Autodesk Inventor part; units mm, degrees
ref_plane "YZ Plane" through (0, 0, 0) normal (1, 0, 0) x (0, 1, 0)
ref_plane "XZ Plane" through (0, 0, 0) normal (0, 1, 0) x (-1, 0, 0)
ref_plane "XY Plane" through (0, 0, 0) normal (0, 0, 1) x (1, 0, 0)
sketch "Эскиз1" plane through (0, 0, 0) normal (0, 1, 0) x (-1, 0, 0)
  line L0 (50, -40) -> (-50, -40)
  line L1 (-50, -40) -> (-50, 40)
  line L2 (-50, 40) -> (50, 40)
  line L3 (50, 40) -> (50, -40)
  line L4 (50, -40) -> (-50, 40) construction
  line L5 (-50, -40) -> (50, 40) construction
  line L6 (21.6, -30) -> (-21.6, -30)
  line L7 (-21.6, -30) -> (-21.6, -6.9)
  line L8 (-21.6, -6.9) -> (21.6, -6.9)
  line L9 (21.6, -6.9) -> (21.6, -30)
  line L10 (-53, -43) -> (53, -43)
  line L11 (53, -43) -> (53, 43)
  line L12 (53, 43) -> (-53, 43)
  line L13 (-53, 43) -> (-53, -43)
  line L14 (53, 43) -> (68, 43)
  line L15 (68, 43) -> (68, -43)
  line L16 (68, -43) -> (53, -43)
  line L17 (53, -43) -> (53, 43)
  line L18 (-53, -43) -> (68, -43)
  line L19 (68, -43) -> (68, 43)
  line L20 (68, 43) -> (-53, 43)
  line L21 (-53, 43) -> (-53, -43)
  line L22 (0, -40) -> (0, 40)
  circle A0 centre (-30, 20) radius 5
  circle A1 centre (-30, 20) radius 7
  line L23 (-30, 20) -> (-30, 40)
  line L24 (-28, 30.5826) -> (-32, 30.5826)
  line L25 (-32, 30.5826) -> (-32, 24.5826)
  line L26 (-32, 24.5826) -> (-28, 24.5826)
  line L27 (-28, 24.5826) -> (-28, 30.5826)
  line L28 (-28, 30.5826) -> (-32, 24.5826) construction
  line L29 (-32, 30.5826) -> (-28, 24.5826) construction
  line L30 (-34, 22.5826) -> (-34, 32.5826)
  line L31 (-34, 32.5826) -> (-26, 32.5826)
  line L32 (-26, 32.5826) -> (-26, 22.5826)
  line L33 (-26, 22.5826) -> (-34, 22.5826)
  line L34 (-28, 30.5826) -> (-32, 30.5826)
  line L35 (-32, 30.5826) -> (-32, 32.5826)
  line L36 (-32, 32.5826) -> (-28, 32.5826)
  line L37 (-28, 32.5826) -> (-28, 30.5826)
  line L38 (-55.5, -45.5) -> (70.5, -45.5)
  line L39 (70.5, -45.5) -> (70.5, 45.5)
  line L40 (-55.5, -45.5) -> (-55.5, 45.5)
  line L41 (-55.5, 45.5) -> (70.5, 45.5)
  point P0 (0, 0)
  point P1 (0, -30)
  point P2 (-30, 27.5826)
  point P3 (53, -43)
  point P4 (-26, 25.7446)
  point P5 (-34, 25.7446)
  point P6 (53, -43)
  dimension "d7" = 10
  dimension "d0" = 100
  dimension "d1" = 80
  dimension "d2" = 43.2
  dimension "d3" = 23.1
  dimension "d4" = 3
  dimension "d5" = 15
  dimension "d6" = 10
  dimension "d8" = 2
  dimension "d9" = 20
  dimension "d10" = 20
  dimension "d11" = 4
  dimension "d12" = 6
  dimension "d13" = 2
  dimension "d22" = 2.5
  dimension "d23" = 2.5
extrude "Выдавливание1" add sketch "Эскиз1" along normal blind 2.5 contours L0 L22 L6 L9 L8 L2 L3 | L0 L1 L2 L22 L8 L7 L6 | L13 L12 L11 L10 | L11 L14 L15 L16 | A0 L30 L33 L32 | L32 L33 L23 L26 A0 | A0 L26 L23 L33 L30 | L26 L23 A0 | A0 L23 A1 L27 | L25 A1 L23 A0 | A0 L23 L26 | A1 L23 L24 L27 | L25 L24 L23 A1 | L24 L23 L31 L37 | L35 L31 L23 L24 | L40 L41 L39 L38
fillet "Сопряжение1" radius 5 4 edges at (26, 1.25, 25.7446) (28, 1.25, 24.5826) (32, 1.25, 24.5826) (34, 1.25, 25.7446)
fillet "Сопряжение2" radius 1 4 edges at (26, 1.25, 32.5826) (28, 1.25, 32.5826) (32, 1.25, 32.5826) (34, 1.25, 32.5826)
sketch "Эскиз2" plane through (0, 0, 0) normal (0, -1, 0) x (1, 0, 0)
  line L0 (-21.6, -30) -> (21.6, -30)
  line L1 (-21.6, -6.9) -> (-21.6, -30)
  line L2 (21.6, -6.9) -> (-21.6, -6.9)
  line L3 (21.6, -30) -> (21.6, -6.9)
  arc A0 (34, 27.9373) -> (35.25, 24.6301) centre (39, 27.9373) ccw
  arc A1 (24.75, 24.6301) -> (35.25, 24.6301) centre (30, 20) ccw
  arc A2 (24.75, 24.6301) -> (26, 27.9373) centre (21, 27.9373) ccw
  line L4 (26, 31.5826) -> (26, 27.9373)
  arc A3 (28, 31.5826) -> (26, 31.5826) centre (27, 31.5826) ccw
  line L5 (28, 27.1414) -> (28, 31.5826)
  arc A4 (26.5, 23.5707) -> (28, 27.1414) centre (23, 27.1414) ccw
  arc A5 (26.5, 23.5707) -> (33.5, 23.5707) centre (30, 20) ccw
  arc A6 (32, 27.1414) -> (33.5, 23.5707) centre (37, 27.1414) ccw
  line L6 (32, 31.5826) -> (32, 27.1414)
  arc A7 (34, 31.5826) -> (32, 31.5826) centre (33, 31.5826) ccw
  line L7 (34, 27.9373) -> (34, 31.5826)
  circle A8 centre (30, 20) radius 2.5
  point P0 (0, 0)
  dimension "d18" = 5
extrude "Выдавливание2" add sketch "Эскиз2" along normal blind 2.5 contours A8
fillet "Сопряжение3" radius 2 1 edges at (27.5, 0, 20)
sketch "Эскиз3" plane through (0, 0, 0) normal (0, -1, 0) x (1, 0, 0)
  arc A0 (34, 27.9373) -> (35.25, 24.6301) centre (39, 27.9373) ccw
  arc A1 (24.75, 24.6301) -> (35.25, 24.6301) centre (30, 20) ccw
  arc A2 (24.75, 24.6301) -> (26, 27.9373) centre (21, 27.9373) ccw
  line L0 (26, 31.5826) -> (26, 27.9373)
  arc A3 (28, 31.5826) -> (26, 31.5826) centre (27, 31.5826) ccw
  line L1 (28, 27.1414) -> (28, 31.5826)
  arc A4 (26.5, 23.5707) -> (28, 27.1414) centre (23, 27.1414) ccw
  arc A5 (26.5, 23.5707) -> (33.5, 23.5707) centre (30, 20) ccw
  arc A6 (32, 27.1414) -> (33.5, 23.5707) centre (37, 27.1414) ccw
  line L2 (32, 31.5826) -> (32, 27.1414)
  arc A7 (34, 31.5826) -> (32, 31.5826) centre (33, 31.5826) ccw
  line L3 (34, 27.9373) -> (34, 31.5826)
  line L4 (-21.6, -30) -> (21.6, -30)
  line L5 (-21.6, -6.9) -> (-21.6, -30)
  line L6 (21.6, -6.9) -> (-21.6, -6.9)
  line L7 (21.6, -30) -> (21.6, -6.9)
  circle A8 centre (30, 20) radius 4.5
  line L8 (55.5, -45.5) -> (-70.5, -45.5)
  line L9 (55.5, 45.5) -> (55.5, -45.5)
  line L10 (-70.5, 45.5) -> (55.5, 45.5)
  line L11 (-70.5, -45.5) -> (-70.5, 45.5)
  arc A9 (34, 27.9373) -> (35.25, 24.6301) centre (39, 27.9373) ccw
  arc A10 (24.75, 24.6301) -> (35.25, 24.6301) centre (30, 20) ccw
  arc A11 (24.75, 24.6301) -> (26, 27.9373) centre (21, 27.9373) ccw
  line L12 (26, 31.5826) -> (26, 27.9373)
  arc A12 (28, 31.5826) -> (26, 31.5826) centre (27, 31.5826) ccw
  line L13 (28, 27.1414) -> (28, 31.5826)
  arc A13 (26.5, 23.5707) -> (28, 27.1414) centre (23, 27.1414) ccw
  arc A14 (26.5, 23.5707) -> (33.5, 23.5707) centre (30, 20) ccw
  arc A15 (32, 27.1414) -> (33.5, 23.5707) centre (37, 27.1414) ccw
  line L14 (32, 31.5826) -> (32, 27.1414)
  arc A16 (34, 31.5826) -> (32, 31.5826) centre (33, 31.5826) ccw
  line L15 (34, 27.9373) -> (34, 31.5826)
  line L16 (-21.6, -30) -> (21.6, -30)
  line L17 (-21.6, -6.9) -> (-21.6, -30)
  line L18 (21.6, -6.9) -> (-21.6, -6.9)
  line L19 (21.6, -30) -> (21.6, -6.9)
  circle A17 centre (30, 20) radius 4.5
  line L20 (53, 43) -> (53, -43)
  line L21 (53, -43) -> (-68, -43)
  line L22 (-68, -43) -> (-68, 43)
  line L23 (-68, 43) -> (53, 43)
  dimension "d28" = 2.5
extrude "Выдавливание3" add sketch "Эскиз3" along normal blind 24.04 contours L8 L11 L10 L9
sketch "Эскиз4" plane through (-70.5, 2.5, -45.5) normal (-1, 0, 0) x (0, 0, 1)
  line L0 (91, -26.54) -> (91, 0)
  line L1 (0, 0) -> (91, 0)
  line L2 (0, -26.54) -> (0, 0)
  line L3 (91, -26.54) -> (0, -26.54)
  line L4 (0, 0) -> (0, -26.54)
  line L5 (0, -13.27) -> (-40, -13.27)
  circle A0 centre (-40, -13.27) radius 40
  line L6 (0, -26.54) -> (0, 0)
  line L7 (0, -26.54) -> (-2.2653, -26.54)
  line L8 (-2.2653, -26.54) -> (-2.2653, 0)
  line L9 (-2.2653, 0) -> (0, 0)
  line L10 (0, 0) -> (0, -26.54)
  line L11 (0, 0) -> (91, 0)
  point P0 (45.5, -2.5)
  point P1 (-2.2653, -26.54)
  dimension "d29" = 80
extrude "Выдавливание4" add sketch "Эскиз4" against normal up to surface (126 mm away) contours L7 A0 L2 | L2 A0 L9
sketch "Эскиз5" plane through (-70.5, -24.04, 45.5) normal (-1, 0, 0) x (0, 0, 1)
  line L0 (0, 0) -> (0, 26.54)
  line L1 (0, 26.54) -> (-93.2653, 26.54)
  arc A0 (-93.2653, 0) -> (-93.2653, 26.54) centre (-131, 13.27) ccw
  line L2 (0, 0) -> (-93.2653, 0)
  circle A1 centre (-131, 13.27) radius 40
  circle A2 centre (-131, 13.27) radius 36
  line L3 (-93.2653, 0) -> (-97.535, 0)
  arc A3 (-93.2653, 0) -> (-93.2653, 26.54) centre (-131, 13.27) ccw
  line L4 (-93.2653, 26.54) -> (-97.535, 26.54)
  point P0 (-45.5, 24.04)
  dimension "d32" = 4
extrude "Выдавливание5" add sketch "Эскиз5" against normal blind 4 contours L3 A2 L4 A0
sketch "Эскиз6" plane through (-70.5, -24.04, 45.5) normal (-1, 0, 0) x (0, 0, 1)
  line L0 (-2.5, 24.04) -> (-88.5, 24.04)
  line L1 (-2.5, 24.04) -> (-2.5, 0)
  line L2 (-88.5, 0) -> (-2.5, 0)
  line L3 (-88.5, 24.04) -> (-88.5, 0)
  line L4 (-88.5, 24.04) -> (-88.5, 0)
  line L5 (-88.5, 12.02) -> (-2.5, 12.02)
  line L6 (-2.5, 24.04) -> (-2.5, 0)
  line L7 (-10.5, 9.27) -> (-80.5, 9.27)
  line L8 (-80.5, 9.27) -> (-80.5, 14.77)
  line L9 (-80.5, 14.77) -> (-10.5, 14.77)
  line L10 (-10.5, 14.77) -> (-10.5, 9.27)
  line L11 (-10.5, 9.27) -> (-80.5, 14.77) construction
  line L12 (-80.5, 9.27) -> (-10.5, 14.77) construction
  point P0 (-45.5, 24.04)
  point P1 (-45.5, 12.02)
  dimension "d35" = 70
  dimension "d36" = 5.5
extrude "Выдавливание6" cut sketch "Эскиз6" against normal blind 4 contours L10 L7 L8 L5 | L5 L8 L9 L10
properties part number "tacho_base"
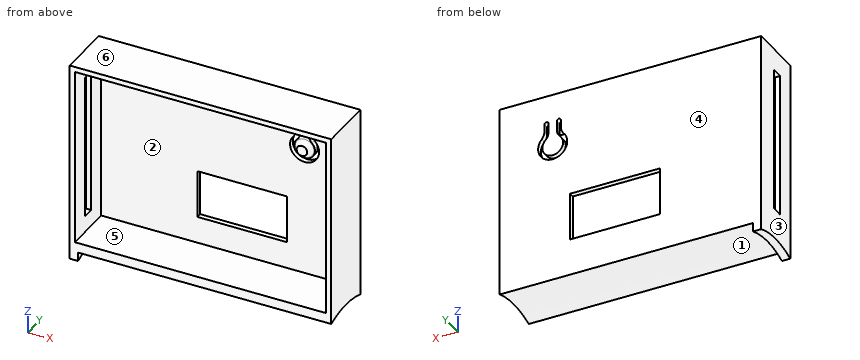
Geometry: final body of the model. Coordinates: model frame, mm. Face numbers are marked on the shaded views. A direction names the side the tool comes from. Round coordinates to 2 decimals unless told otherwise and drop trailing zeros. Order: outer loops, then holes, each group sorted by start corner. A loop starts at its lowest first (then second) coordinate and runs counter-clockwise, first axis right, second up. Notation, with made-up numbers: (83.25, -29) - (119.25, -29) arc R5 ccw to (119.25, -23) - close; hole circle Ø2 at (0, 84). An arc over 180 degrees is marked (long way). Use CSV: the item, a comma, the result in double quotes. Start each with the question number.
Q1. Section query A-A (z = 20). Return loops of the section in (x, y), and give its area (3 significant figures).
Q2. Section query D-D (y = -5.5). Return loops of the section in (x, z).
Q3. Material intervals for line 1 along X through (y, z) = (1.65, 20); line 2 along X through (y, z) = (-20.25, -11); line 3 along Z through (x, y) = (38.5, -11.25), sorted ascending. Write a range as from..to.
Q4. Access query for the marked faces 1, 2 and 3. Directions: +Z, -Z, +X, -X, +Y, -Y. A direction counts if a zero-diameter tool reaches every point of the face in a straight line with its end or side. Return the directions, or none.
Q5. Section query B-B (z = -22.5). Return loops of the section in (x, y).
Q6. First-contact query: pin 1 (3.5 mm diameter, centred on y = -6, z = -50, fed in from +X); pin 2 (10 mm diameter, centred on x = 39.5, z = -14.5, fed in from -Y); pin 3 (18 mm diameter, centred on x = 30, z = 20, fed in from -Y). Flat tips, straight axial feed; report the tip coordinate or a pass-through.
Q7. Mould query, pull axis Z, two halves, no side actions, for the marked faces 4, 5 and 6. Classes: +Z half, -Z half, draft (parallel to the pull), parting line (faces both ways), or undercut.
Q8. Section query C-C (x = 30). Return loops of the section in (y, z), and give its area (3 significant figures).
Result set:
1,outline,"(-70.5, -24.04) - (-68, -24.04) - (-68, -14.77) - (-70.5, -14.77) - close; (-70.5, -9.27) - (-68, -9.27) - (-68, 0) - (23, 0) - (23, 2.5) - (-70.5, 2.5) - close; (25, 0) - (25.5, 0) arc R2 cw to (27.5, -2) - (27.5, -2.5) - (32.5, -2.5) - (32.5, -2) arc R2 cw to (34.5, 0) - (35, 0) - (35, 2.5) - (25, 2.5) - close; (37, 0) - (53, 0) - (53, -24.04) - (55.5, -24.04) - (55.5, 2.5) - (37, 2.5) - close"
1,area,"426 mm2"
2,outline,"(-70.5, -49.89) - (-66.5, -49.89) - (-66.5, -45.85) - (55.5, -45.85) - (55.5, 45.5) - (-70.5, 45.5) - close; hole (-68, -43) - (53, -43) - (53, 43) - (-68, 43) - close"
3,line 1,"x = -70.5..23, 25..35, 37..55.5"
3,line 2,"x = -70.5..-68, 53..55.5"
3,line 3,"z = -45.5..-43, 43..45.5"
4,face 1,"-Z, +X"
4,face 2,"-Y"
4,face 3,"+Z, -Z, -X, +Y, -Y"
5,outline,"(-70.5, -24.04) - (-68, -24.04) - (-68, -14.77) - (-70.5, -14.77) - close; (-70.5, -9.27) - (-68, -9.27) - (-68, 0) - (-21.6, 0) - (-21.6, 2.5) - (-70.5, 2.5) - close; (21.6, 0) - (53, 0) - (53, -24.04) - (55.5, -24.04) - (55.5, 2.5) - (21.6, 2.5) - close"
6,pin 1,"stops at x = -66.5"
6,pin 2,"stops at y = 0"
6,pin 3,"stops at y = -2.5"
7,face 4,"draft"
7,face 5,"undercut"
7,face 6,"+Z half"
8,outline,"(-24.04, -47.77) arc R40 cw to (2.5, -47.77) - (2.5, 13) - (0, 13) - (0, -43) - (-24.04, -43) - close; (-24.04, 43) - (0, 43) - (0, 24.5) arc R2 cw to (-2, 22.5) - (-2.5, 22.5) - (-2.5, 17.5) - (-2, 17.5) arc R2 cw to (0, 15.5) - (0, 15) - (2.5, 15) - (2.5, 45.5) - (-24.04, 45.5) - close"
8,area,"377 mm2"
